Work out the finished part from the listing and answer in its coordinate system (mm). A direction names the side the tool comes from. Coordinates: 2 decimals unless noted, no trailing zeros. Write each loop counter-clockwise with the first axis right and the second up, starting at its lowest first coordinate (ties: lowest second). Pieces come first, ordered by that corner, then holes. Notation, with made-up numbers: M 4,-33 L 18,-33 A25 cw 18,5 Z; hole C 85.5,-29 d2. An arc over 180 degrees is marked long. Answer as CSV lines item,"result". Start each with the question number.
(1) Flat-ended cylindrical pins translate along their axes: P1, Ø2, axis at x = -3.5, y = -1, coming from the -Z side; P2, Ø1.9, axis at y = -0.5, z = -22, coming from the -X side; P3, Ø1.5, axis at x = 27, y = -2, coming from the +Z side. Find the tip coordinate at first contact, or state that the pin passes through.
(2) A cutting plane is placed at C-C on x = -10. Give the vertices of the cut face in (y, z) (3 decimals).
(3) A cutting plane is placed at D-D on z = -21. Give the vertices of the cut face in (x, y) (3 decimals).
(4) The mould has two halves that part along Z. Classify faces 1 (the flat face through (-7.676, 0.044, -13.848)), 2 (the flat face through (-6.2, 0, -21)), 3 (the flat face through (6.2, 0, -21)), 4 (the cylindrical face through (22.498, 0.044, -62.765)): released by +Z, released by -Z, zero draft, split by the parting line, or undercut.
(5) Find the intervals of material crossed by L1, parallel to Z at x = -3, y = -1; L2, parallel to X at y = -0.5, z = -44; L3, parallel to Z at x = -1, y = -1.5, in increasing order. Write a range as [from, to].
(6) A cutting plane is placed at A-A on y = 1.5. Give the vertices of the cut face in (x, z) (3 decimals).
(7) A cutting plane is placed at B-B on z = -44.5. Give the vertices of the cut face in (x, y) (3 decimals).
(8) For faces 5 (the cylindrical face through (-7.59, 0.04, -31.46)), 6 (the cylindrical face through (7.677, 0.044, -17.216)), 7 (the cylindrical face through (18.71, 0.04, -50.63)), determine the directions among +Z, -Z, +X, -X, +Y, -Y from which every point of the face is accessible in a straight line to the end or side of a thin tool.
from build123d import *

# Parameters (mm, degrees)
BOSS_EXTRUDE1_DEPTH = 3.175


with BuildPart() as part:
    # Sketch8 → Boss-Extrude1 (new, symmetric)
    with BuildSketch(Plane(origin=(0, 0, 0), x_dir=(1, 0, 0), z_dir=(0, 1, 0))):
        with BuildLine():
            Line((-6.254044101, 11.282594222), (-9.138661342, 16.48658148))
            ThreePointArc((-9.138661342, 16.48658148), (-7.69744661, 17.206737508), (-6.2, 17.80119378))
            Line((-6.2, 17.80119378), (-6.2, 24.631686909))
            ThreePointArc((-6.2, 24.631686909), (-7.626220631, 31.546787733), (-11.672110257, 37.333280783))
            ThreePointArc((-11.672110257, 37.333280783), (-15.789036104, 55.963427524), (0, 66.675))
            ThreePointArc((0, 66.675), (22.804193056, 62.654005491), (42.857863876, 51.076013245))
            ThreePointArc((42.857863876, 51.076013245), (43.640544768, 42.12992971), (34.694461233, 41.347248817))
            ThreePointArc((34.694461233, 41.347248817), (18.460537236, 50.719909207), (0, 53.975))
            ThreePointArc((0, 53.975), (-3.988447659, 51.269163755), (-2.948476431, 46.563026873))
            ThreePointArc((-2.948476431, 46.563026873), (4.019706834, 36.595971198), (6.2, 24.631686909))
            Line((6.2, 24.631686909), (6.2, 17.80119378))
            ThreePointArc((6.2, 17.80119378), (7.69744661, 17.206737508), (9.138661342, 16.48658148))
            Line((9.138661342, 16.48658148), (6.254044101, 11.282594222))
            ThreePointArc((6.254044101, 11.282594222), (0, 12.9), (-6.254044101, 11.282594222))
        make_face()
    extrude(amount=BOSS_EXTRUDE1_DEPTH, both=True)


solid = part.part
Here are the results:
1,P1,"stops at z = -66.49"
1,P2,"stops at x = -6.2"
1,P3,"stops at z = -46.3"
2,outline,"M -3.175,-63.421 L 3.175,-63.421 L 3.175,-35.512 L -3.175,-35.512 Z"
3,outline,"M -6.2,-3.175 L 6.2,-3.175 L 6.2,3.175 L -6.2,3.175 Z"
4,face 1,"released by +Z"
4,face 2,"undercut"
4,face 3,"undercut"
4,face 4,"released by -Z"
5,L1,"z = [-66.41, -52.75], [-46.61, -12.55]"
5,L2,"x = [-16.01, -0.5], [31.26, 44.73]"
5,L3,"z = [-66.65, -53.86], [-44.58, -12.86]"
6,outline,"M -11.672,-37.333 A16.992 ccw 0,-66.675 A66.675 ccw 42.858,-51.076 A6.35 ccw 34.694,-41.347 A53.975 cw 0,-53.975 A4.292 cw -2.948,-46.563 A28.509 ccw 6.2,-24.632 L 6.2,-17.801 A18.85 ccw 9.139,-16.487 L 6.254,-11.283 A12.9 cw -6.254,-11.283 L -9.139,-16.487 A18.85 ccw -6.2,-17.801 L -6.2,-24.632 A17.477 cw Z"
7,outline,"M -16.183,-3.175 L -0.93,-3.175 L -0.93,3.175 L -16.183,3.175 Z; M 30.546,-3.175 L 44.891,-3.175 L 44.891,3.175 L 30.546,3.175 Z"
8,face 5,"-X, +Y, -Y"
8,face 6,"+X, +Y, -Y"
8,face 7,"+Y, -Y"
